from build123d import *

# Parameters (mm, degrees)
EXTRUDE_1_DEPTH     = 20
SKETCH_2_R          = 2.75
CUT_EXTRUDE_1_DEPTH = 40.770397535
SKETCH_3_W          = 5
SKETCH_3_H          = 20
EXTRUDE_2_DEPTH     = 15
SKETCH_4_R          = 2.75
CUT_EXTRUDE_2_DEPTH = 41.757009157
FILLET_1_R          = 2
SKETCH_5_R          = 4
CUT_EXTRUDE_3_DEPTH = 2


with BuildPart() as part:
    # 草图1 → 凸台-拉伸1 (new body)
    with BuildSketch(Plane(origin=(0, 0, 0), x_dir=(1, 0, 0), z_dir=(0, 1, 0))):
        Polygon((-12.057971014, 6.222222222), (19.942028986, 6.222222222), (19.942028986, -21.777777778), (14.942028986, -21.777777778), (14.942028986, -16.777777778), (14.942028986, 1.222222222), (-7.057971014, 1.222222222), (-7.057971014, -16.777777778), (-7.057971014, -21.777777778), (-12.057971014, -21.777777778), align=None)
    extrude(amount=EXTRUDE_1_DEPTH)

    # 草图2 → 切除-拉伸1 (cut, through all)
    with BuildSketch(Plane(origin=(0, 0, -6.222222222), x_dir=(-1, 0, 0), z_dir=(0, 0, -1))):
        with Locations((-3.942028986, 10)):
            Circle(SKETCH_2_R)
    extrude(amount=-CUT_EXTRUDE_1_DEPTH, mode=Mode.SUBTRACT)

    # 草图3 → 凸台-拉伸2 (add)
    with BuildSketch(Plane.ZY.offset(12.057971014)):
        with Locations((19.277777778, 10)):
            Rectangle(SKETCH_3_W, SKETCH_3_H)
    extrude_2 = extrude(amount=EXTRUDE_2_DEPTH)

    # 草图4 → 切除-拉伸2 (cut, through all)
    with BuildSketch(Plane(origin=(0, 0, 16.777777778), x_dir=(-1, 0, 0), z_dir=(0, 0, -1))):
        with Locations((19.557971014, 10)):
            Circle(SKETCH_4_R)
    cut_extrude_2 = extrude(amount=-CUT_EXTRUDE_2_DEPTH, mode=Mode.SUBTRACT)

    # 镜向5: 凸台-拉伸2, 切除-拉伸2 across plane
    add(extrude_2.mirror(Plane.ZY.offset(-3.942028986)))
    add(cut_extrude_2.mirror(Plane.ZY.offset(-3.942028986)), mode=Mode.SUBTRACT)

    # 圆角1
    fillet_1_edges = [part.edges().sort_by_distance(p)[0] for p in [
        (-12.057971014, 10, -6.222222222),
        (19.942028986, 10, -6.222222222),
        (-27.057971014, 0, 19.277777778),
        (-27.057971014, 20, 19.277777778),
        (34.942028986, 0, 19.277777778),
        (34.942028986, 20, 19.277777778),
    ]]
    fillet(fillet_1_edges, radius=FILLET_1_R)

    # 草图5 → 切除-拉伸3 (cut)
    with BuildSketch(Plane(origin=(0, 0, -6.222222222), x_dir=(-1, 0, 0), z_dir=(0, 0, -1))):
        with Locations((-3.942028986, 10)):
            Circle(SKETCH_5_R)
    extrude(amount=-CUT_EXTRUDE_3_DEPTH, mode=Mode.SUBTRACT)


solid = part.part
The model under review builds one solid part; all positions refer to its coordinate system, in mm. A direction names the side the tool comes from. Give positions to 0.01 mm unless a question says otherwise; leave off trailing zeros. Loops run counter-clockwise (first coordinate to the right, second up) from the corner with the lowest first, then second, coordinate; pieces in that order, holes last. Notation, with made-up numbers: (-34.5, 89.25) -> (2.5, 89.25) arc R26 cw to (2.5, 123.25) -> close; hole circle Ø1 at (-13.75, 84.25). An arc over 180 degrees is marked (long way). Put each result on its own line as item: value. Start each with the question number.
1. Wall thickness on probe 1 along X at (y, z) = (5.25, 7.25); probe 2 along Z at (x, y) = (8, 8); probe 3 along X at (y, z) = (1, 17.5): over which ranges is each line inside the solid? List them lowest first.
2. Mouldability with a two-part tool opening along Y and no side actions: class faces 1 (the face through (19.37, 10.14, -5.62)), 2 (the face through (27.084, 12.727, 19.243)), 3 (the face through (4, 20, -2)) as released by +Y, released by -Y, zero draft, split by the parting line, or undercut.
3. Clearance check with flat-ended pins moving along their axes: P1, Ø5, axis at x = 11.5, y = 10, coming from the +Z side; P2, Ø6, axis at y = 11, z = 12, coming from the +X side; P3, Ø1, axis at y = 6.5, z = 15.5, coming from the -X side; P4, Ø5, axis at y = 11.5, z = 16, coming from the +X side. State where each tip first meets the part, or that it passes through.
4. We need section B-B on y = 10. State how many separate pieces and enclosed holes the cut face has, then the cut area to 3 significant figures.
5. We need section A-A on z = 18.5. State the section outline as (x, y) points.
6. We need section D-D on x = -18. State the section outline as (y, z) points, then the cut area to 3 significant figures.
7. For faces 4 (the face through (-12.058, 10, 6)), 5 (the face through (19.942, 10, 6)), 6 (the face through (34.37, 19.4, 19.31)), 7 (the face through (14.942, 10, 10)), 8 (the face through (5, 7, -4.222)), list the 3-axis set-ups (+Z, -Z, +X, -X, +Y, -Y) from which the entire face can be reached by the end or side of a thin tool; tool diameter is ignored.
8. We need section C-C on z = 7.5. State the section outline as (x, y) points.
Determined:
1. probe 1: -12.06 to -7.06, 14.94 to 19.94
1. probe 2: -6.22 to -1.22
1. probe 3: -26.79 to -7.06, 14.94 to 34.67
2. face 1: zero draft
2. face 2: undercut
2. face 3: released by +Y
3. P1: z = -1.22
3. P2: x = 19.94
3. P3: x = -12.06
3. P4: x = 34.94
4. separate pieces: 4
4. enclosed holes: 0
4. area: 451 mm^2
5. outline: (-27.06, 2) arc R2 ccw to (-25.06, 0) -> (-7.06, 0) -> (-7.06, 20) -> (-25.06, 20) arc R2 ccw to (-27.06, 18) -> close; (14.94, 0) -> (32.94, 0) arc R2 ccw to (34.94, 2) -> (34.94, 18) arc R2 ccw to (32.94, 20) -> (14.94, 20) -> close; hole circle Ø5.5 at (-19.56, 10); hole circle Ø5.5 at (27.44, 10)
6. outline: (0, 16.78) -> (7.73, 16.78) -> (7.73, 21.78) -> (0, 21.78) -> close; (12.27, 16.78) -> (20, 16.78) -> (20, 21.78) -> (12.27, 21.78) -> close
6. area: 77.3 mm^2
7. face 4: -Z, -X, +Y, -Y
7. face 5: -Z, +X, +Y, -Y
7. face 6: +Z, -Z, +X, +Y
7. face 7: +Z, +Y, -Y
7. face 8: -Z
8. outline: (-12.06, 0) -> (-7.06, 0) -> (-7.06, 20) -> (-12.06, 20) -> close; (14.94, 0) -> (19.94, 0) -> (19.94, 20) -> (14.94, 20) -> close
